from build123d import *

# Parameters (mm, degrees)
F1_DEPTH     = 20
F2_DEPTH     = 12.5
F3_DEPTH     = 5
F4_R         = 2
F5_T         = 10
F5_T3_DEPTH  = 29.9026188965
F5_T5_DEPTH  = 27.5
F5_T7_DEPTH  = 27.5
F5_T9_DEPTH  = 29
F5_T11_DEPTH = 45
F5_T13_DEPTH = 29.9026188965
F5_T15_DEPTH = 30


# Not quite as in the source:
# - ends of sketch curves that miss each other by under 0.0002 mm in the source are joined
# - a shell that OpenCascade refuses in one call is made with other operations: the cavity is built on its own and cut out


with BuildPart() as f1:
    # F0 (on Front) → F1 (new body, symmetric)
    with BuildSketch(Plane.XZ):
        Polygon((-98.8679975982, 54.1129348578), (-128.8679975982, 54.1129348578), (-128.8679975982, 24.1129348578), (-98.8679975982, 24.1129348578), (-98.8679975982, 34.0155537543), (-98.8679975982, 43.0155537543), align=None)
    extrude(amount=F1_DEPTH, both=True)

    # F0 (on Front) → F2 (join, symmetric)
    with BuildSketch(Plane.XZ):
        with BuildLine():
            Line((-80.6820849815, 43.0155537543), (-98.8679975982, 43.0155537543))
            Line((-98.8679975982, 43.0155537543), (-98.8679975982, 34.0155537543))
            Line((-98.8679975982, 34.0155537543), (-88.9653787017, 34.0155537543))
            Line((-88.9653787017, 34.0155537543), (-80.682094855, 34.0155537543))
            add(Edge.make_bspline(
                [(-80.682094855, 34.0155537543), (-66.1309954288, 34.0155509655), (-57.1216260093, 40.1806794107), (-55.0665845173, 50.5349263549)],
                knots=[0, 0, 0, 0, 30.4802237684, 30.4802237684, 30.4802237684, 30.4802237684], degree=3))
            Line((-55.0665845173, 50.5349263549), (-64.3839240074, 50.5349263549))
            add(Edge.make_bspline(
                [(-80.6820849815, 43.0155537543), (-79.1809668737, 43.0155537553), (-76.3999490421, 43.1750788515), (-72.9213473732, 43.8149397212), (-70.1430488739, 44.758463036), (-68.0271542887, 45.9005167962), (-66.4709613794, 47.1632066722), (-65.3230275472, 48.5510213805), (-64.6991129712, 49.71943479), (-64.4207731634, 50.4356187157), (-64.3839240074, 50.5349263549)],
                knots=[2.262e-07, 2.262e-07, 2.262e-07, 2.262e-07, 0.125, 0.25, 0.375, 0.5, 0.625, 0.75, 0.875, 0.8947169283, 0.8947169283, 0.8947169283, 0.8947169283], degree=3))
        make_face()
    extrude(amount=F2_DEPTH, both=True)

    # F0 (on Front) → F3 (join, symmetric)
    with BuildSketch(Plane.XZ):
        Polygon((-98.8679975982, 34.0155537543), (-98.8679975982, 24.1129348578), (-88.9653787017, 34.0155537543), align=None)
    extrude(amount=F3_DEPTH, both=True)

    # F4
    f4_edges = [f1.edges().sort_by_distance(p)[0] for p in [
        (-98.867998, -20, 39.112935),
        (-128.867998, -20, 39.112935),
        (-98.867998, 20, 39.112935),
        (-128.867998, 20, 39.112935),
    ]]
    fillet(f4_edges, radius=F4_R)

    # F5: shell of thickness 10, made by hand


with BuildPart() as f5_core1:
    # F5_t2: copy of F1
    add(f1.part)

    # the walls: a layer under each face that stays
    f5_faces = [f5_core1.faces().sort_by_distance(p)[0] for p in [
        (-113.8679975982, 20, 39.1129348578),
        (-98.8679975982, 12, 29.1129348578),
        (-128.8679975982, 0, 39.1129348578),
        (-113.8679975982, -20, 39.1129348578),
        (-113.8679975982, 0, 24.1129348578),
        (-97.2175611154, -5, 29.0642443061),
        (-97.2175611154, 5, 29.0642443061),
        (-95.8370138076, 8.3333333333, 34.0155537543),
        (-76.9672910577, -12.5, 42.2752386602),
        (-76.9672910577, 12.5, 42.2752386602),
        (-89.7750412898, 0, 43.0155537543),
        (-93.9166881499, 0, 29.0642443061),
        (-63.1883179608, -6.25, 38.3923964047),
        (-63.1883179608, 6.25, 38.3923964047),
        (-59.7252542624, 0, 50.5349263549),
        (-68.9445639905, -6.25, 45.4259334498),
        (-68.9445639905, 6.25, 45.4259334498),
    ]]
    thicken(f5_faces, amount=-F5_T, mode=Mode.SUBTRACT)

    # F5_s4 → F5_t3 (cut)
    with BuildSketch(Plane.XY.offset(14.1129348578)):
        Polygon((-98.7679975982, -5.1), (-108.8679975982, -5), (-108.8679975982, 5), (-98.8679975982, 5), align=None)
        Polygon((-98.7679975982, 5.1), (-108.8679975982, 5), (-108.8679975982, -5), (-98.8679975982, -5), align=None)
    extrude(amount=F5_T3_DEPTH, mode=Mode.SUBTRACT)

    # F5_s6 → F5_t5 (cut)
    with BuildSketch(Plane.XZ.offset(-5)):
        Polygon((-98.7679975982, 33.9155537543), (-108.8679975982, 34.0155537543), (-108.8679975982, 44.0155537543), (-98.8679975982, 44.0155537543), align=None)
    extrude(amount=F5_T5_DEPTH, mode=Mode.SUBTRACT)

    # F5_s8 → F5_t7 (cut)
    with BuildSketch(Plane.XZ.offset(-22.5)):
        Polygon((-98.7679975982, 33.9155537543), (-108.8679975982, 34.0155537543), (-108.8679975982, 44.0155537543), (-98.8679975982, 44.0155537543), align=None)
    extrude(amount=F5_T7_DEPTH, mode=Mode.SUBTRACT)

    # F5_s10 → F5_t9 (cut)
    with BuildSketch(Plane.XY.offset(24.0155537543)):
        Polygon((-98.7679975982, -12.6), (-108.8679975982, -12.5), (-108.8679975982, -2.5), (-98.8679975982, -2.5), align=None)
        Polygon((-98.7679975982, 12.6), (-108.8679975982, 12.5), (-108.8679975982, 2.5), (-98.8679975982, 2.5), align=None)
    extrude(amount=F5_T9_DEPTH, mode=Mode.SUBTRACT)

    # F5_s12 → F5_t11 (cut)
    with BuildSketch(Plane.XZ.offset(-22.5)):
        Polygon((-98.7679975982, 43.1155537543), (-108.8679975982, 43.0155537543), (-108.8679975982, 33.0155537543), (-98.8679975982, 33.0155537543), align=None)
    extrude(amount=F5_T11_DEPTH, mode=Mode.SUBTRACT)

    # F5_s14 → F5_t13 (cut)
    with BuildSketch(Plane.YZ.offset(-108.8679975982)):
        Polygon((-5.1, 33.9155537543), (5, 34.0155537543), (5, 44.0155537543), (-5, 44.0155537543), align=None)
        Polygon((5.1, 33.9155537543), (-5, 34.0155537543), (-5, 44.0155537543), (5, 44.0155537543), align=None)
    extrude(amount=F5_T13_DEPTH, mode=Mode.SUBTRACT)

    # F5_s16 → F5_t15 (cut)
    with BuildSketch(Plane.XZ.offset(-15)):
        Polygon((-88.8946680236, 33.8448430762), (-88.9653787017, 44.0155537543), (-93.1075143254, 44.0155537543), (-96.0364465136, 41.0866215662), align=None)
    extrude(amount=F5_T15_DEPTH, mode=Mode.SUBTRACT)


with BuildPart() as f1_1:
    add(f1.part)

    # what is left inside the walls is the cavity
    f5_cavity = [f5_core1.part.solids().sort_by_distance(p)[0] for p in [
        (-118.767998, 3.333333, 44.112935),
    ]]
    add(f5_cavity, mode=Mode.SUBTRACT)


solid = f1_1.part
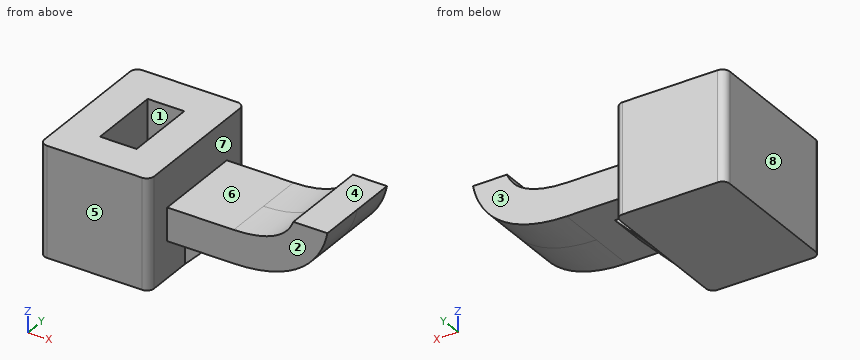
The listing builds one solid part. Answer for the finished solid, in the listing's coordinates (mm). Face numbers are marked on the shaded views. A direction names the side the tool comes from. Round coordinates to 2 decimals unless told otherwise and drop trailing zeros. Write each loop counter-clockwise with the first axis right and the second up, starting at its lowest first coordinate (ties: lowest second). Pieces come first, ordered by that corner, then holes. Notation, with made-up numbers: M 89.25,50.5 L 143.25,50.5 A20 cw 143.25,86.5 Z; hole C 22,-19 d1. An arc over 180 degrees is marked long. Write each question's results on one line, items separated by ' | '. Start each with the question number.
(1) Find the intervals of material crossed by line 1 (Y direction, x = -118, z = 48); line 2 (X direction, y = 7, z = 46.5); line 3 (X direction, y = -2, z = 49.5), in increasing order.
(2) The part is cut by section B-B, the plane z = 46.75. Give the number of separate pieces and of enclosed holes in the cut face, and give its area (3 significant figures).
(3) The part is cut by section A-A, the plane x = -115.5. Write down the section's boundary in (y, z), and give its area (3 significant figures).
(4) Each of these flat-tipped pins is pushed along its axis until it touches: P1, Ø1, axis at y = -12, z = 38, coming from the +X side; P2, Ø5, axis at x = -78.5, z = 39, coming from the -Y side; P3, Ø5, axis at x = -94, z = 29, coming from the +Y side. Where does it stop, or does it pass through?
(5) The part is cut by section D-D, the plane z = 27.75. Write down the section's boundary in (x, y).
(6) For the marked faces 1, 2, 3 and 4, determine the directions among +Z, -Z, +X, -X, +Y, -Y from which every point of the face is accessible in a straight line to the end or side of a thin tool.
(7) Determine the mould class of the marked faces 5, 6, 7 and 8 for opening direction X: +X half, -X half, draft (parallel to the pull), parting line (faces both ways), or undercut.
(8) The part is cut by section C-C, the plane y = -14. Write down the section's boundary in (x, z), and give its area (3 significant figures).
Worked answers:
1) line 1: y = -20 to -10, 10 to 20 | line 2: x = -128.87 to -118.87, -108.87 to -98.87, -67.32 to -56.31 | line 3: x = -128.87 to -118.87, -108.87 to -98.87, -64.84 to -55.3
2) separate pieces: 2 | enclosed holes: 1 | area: 1,270 mm²
3) outline: M -20,24.11 L 20,24.11 L 20,54.11 L 10,54.11 L 10,34.11 L -10,34.11 L -10,54.11 L -20,54.11 Z | area: 800 mm²
4) P1: stops at x = -63.03 | P2: stops at y = -12.5 | P3: stops at y = 5
5) outline: M -128.87,-18 A2 ccw -126.87,-20 L -100.87,-20 A2 ccw -98.87,-18 L -98.87,-5 L -95.23,-5 L -95.23,5 L -98.87,5 L -98.87,18 A2 ccw -100.87,20 L -126.87,20 A2 ccw -128.87,18 Z
6) face 1: +Z | face 2: +Z, -Z, +X, -Y | face 3: +Z, -Z, +X, +Y | face 4: +Z, +X, +Y, -Y
7) face 5: draft | face 6: undercut | face 7: undercut | face 8: -X half
8) outline: M -128.87,24.11 L -98.87,24.11 L -98.87,54.11 L -128.87,54.11 Z | area: 900 mm²
